Geometry: final body of the model. Coordinates: model frame, mm. Face numbers are marked on the shaded views. Give positions to 0.01 mm unless a question says otherwise; leave off trailing zeros. Write each loop counter-clockwise with the first axis right and the second up, starting at its lowest first coordinate (ties: lowest second). Pieces come first, ordered by that corner, then holes. Notation, with made-up numbers: M 82,-15.5 L 105,-15.5 A15 ccw 105,5.5 Z; hole C 6.25,42.25 d10. An arc over 180 degrees is marked long. Answer as a JSON object with one key per item and string values.
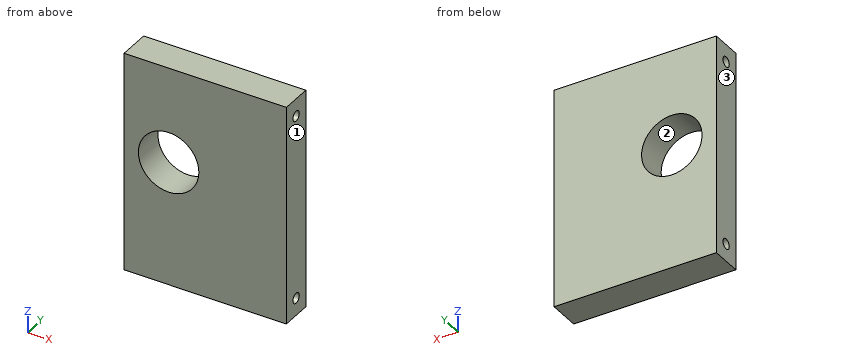
from build123d import *

# Parameters (mm, degrees)
SKETCH_1_W          = 25.5
SKETCH_1_H          = 34.5
EXTRUDE_1_DEPTH     = 5
M2X0_4_1_AT_2_COUNT = 2
M2X0_4_1_AT_2_PITCH = 29
SKETCH_4_R          = 4.75
CUT_EXTRUDE_1_DEPTH = 23.025553342


with BuildPart() as part:
    # 草图1 → 凸台-拉伸1 (new body)
    with BuildSketch(Plane(origin=(0, 0, 0), x_dir=(1, 0, 0), z_dir=(0, 1, 0))):
        Rectangle(SKETCH_1_W, SKETCH_1_H)
    extrude(amount=EXTRUDE_1_DEPTH)

    # 草图3 → M2x0.4 螺纹孔1 (revolve, cut)
    with BuildSketch(Plane(origin=(12.75, 2.5, -14.5), x_dir=(0, 0, -1), z_dir=(0, 1, 0))):
        Polygon((0, 0), (0, 5.680688495), (0.8, 5.2), (0.8, 0), align=None)
    m2x0_4_1 = revolve(axis=Axis((19.1, 2.5, -14.5), (-1, 0, 0)), mode=Mode.SUBTRACT)

    # M2x0.4 螺纹孔1 at 2: M2x0.4 螺纹孔1 ×2
    with Locations(*[(0, 0, i * M2X0_4_1_AT_2_PITCH) for i in range(1, M2X0_4_1_AT_2_COUNT)]):
        add(m2x0_4_1, mode=Mode.SUBTRACT)

    # 镜向1: M2x0.4 螺纹孔1 across plane
    add(m2x0_4_1.mirror(Plane(origin=(0, 0, 0), x_dir=(0, 0, 1), z_dir=(1, 0, 0))), mode=Mode.SUBTRACT)

    # 镜向1 copy 1 sketch → 镜向1 copy 1 (revolve, cut)
    with BuildSketch(Plane(origin=(-12.75, 2.5, 14.5), x_dir=(0, 0, -1), z_dir=(0, 1, 0))):
        Polygon((0, 0), (0, -5.680688495), (0.8, -5.2), (0.8, 0), align=None)
    revolve(axis=Axis((-19.1, 2.5, 14.5), (-1, 0, 0)), mode=Mode.SUBTRACT)

    # 草图4 → 切除-拉伸1 (cut, through all)
    with BuildSketch(Plane.XZ):
        with Locations(Location((-5.75, 2.25, 0), (0, 0, 270))):
            Circle(SKETCH_4_R)
    extrude(amount=-CUT_EXTRUDE_1_DEPTH, mode=Mode.SUBTRACT)


solid = part.part
1) Cut plane B-B on z = 2.25. Return loops of the section in (x, y).
Geometry check:
{"outline": "M -12.75,0 L -10.5,0 L -10.5,5 L -12.75,5 Z; M -1,0 L 12.75,0 L 12.75,5 L -1,5 Z"}
2) Line query: line 1 (Z direction, x = -10.6, y = 2.5); line 2 (Y direction, x = 10.35, z = -14.5); line 3 (Z direction, x = -5.5, y = 2.75). Output: solid intervals per line, ascending. Write a range as from..to.
Geometry check:
{"line 1": "z = -17.25..-15.3, -13.7..13.7, 15.3..17.25", "line 2": "y = 0..1.7, 3.3..5", "line 3": "z = -17.25..-2.49, 6.99..17.25"}
3) Cut plane C-C on y = 1.25. Return loops of the section in (x, z).
Geometry check:
{"outline": "M -12.75,-17.25 L 12.75,-17.25 L 12.75,17.25 L -12.75,17.25 Z; hole C -5.75,2.25 d9.5"}
4) Cut plane A-A on x = 8. Return loops of the section in (y, z).
Geometry check:
{"outline": "M 0,-17.25 L 5,-17.25 L 5,17.25 L 0,17.25 Z; hole C 2.5,-14.5 d1.6; hole C 2.5,14.5 d1.6"}
5) Contact query for flat-ended pins moving along their axis: P1, Ø2.5, axis at y = 2.5, z = -14.5, coming from the +X side; P2, Ø1.3, axis at y = 2.5, z = 14.5, coming from the +X side. Output: stop coordinate, or through.
Geometry check:
{"P1": "stops at x = 12.75", "P2": "stops at x = 7.46"}
6) Pull-direction query (X, two-part tool) for the marked faces 1, 2 and 3; classes: pulls with the +X half, pulls with the -X half, needs draft (parallel to the pull), parting line crosses it, or undercut.
Geometry check:
{"face 1": "pulls with the +X half", "face 2": "undercut", "face 3": "pulls with the -X half"}
